Check sheet for the modelled part. Datum: model origin and axes. Units: mm. A direction names the side the tool comes from. Coordinates: 2 decimals unless noted, no trailing zeros. Order: outer loops, then holes, each group sorted by start corner. A loop starts at its lowest first (then second) coordinate and runs counter-clockwise, first axis right, second up. Notation, with made-up numbers: M 17.25,35.25 L 25.25,35.25 A19 cw 25.25,69.25 Z; hole C 36,16.25 d5. An arc over 180 degrees is marked long. Answer in a Markdown table with one row per item. Add a question column.
from build123d import *

# Parameters (mm, degrees)
SKETCH1_R                = 152.4
SKETCH1_R_2              = 133.35
BOSS_EXTRUDE1_DEPTH      = 38.1
SKETCH2_R                = 152.4
SKETCH2_R_2              = 139.7
CUT_EXTRUDE1_DEPTH       = 31.75
BOSS_EXTRUDE2_DEPTH      = 38.1
FILLET1_R                = 2.54
HOLE1_D                  = 8
HOLE1_DEPTH              = 81.182271537
CIRPATTERN1_COUNT        = 3
FILLET1_OF_CIRPATTERN1_R = 2.54
CIRPATTERN2_COUNT        = 16


with BuildPart() as part:
    # Sketch1 → Boss-Extrude1 (new body)
    with BuildSketch(Plane(origin=(0, 0, 0), x_dir=(1, 0, 0), z_dir=(0, 1, 0))):
        Circle(SKETCH1_R)
        Circle(SKETCH1_R_2, mode=Mode.SUBTRACT)
    extrude(amount=BOSS_EXTRUDE1_DEPTH)

    # Sketch2 → Cut-Extrude1 (cut)
    with BuildSketch(Plane(origin=(0, 38.1, 0), x_dir=(1, 0, 0), z_dir=(0, 1, 0))):
        Circle(SKETCH2_R)
        Circle(SKETCH2_R_2, mode=Mode.SUBTRACT)
    extrude(amount=-CUT_EXTRUDE1_DEPTH, mode=Mode.SUBTRACT)

    # Sketch3 → Boss-Extrude2 (add, through all)
    with BuildSketch(Plane(origin=(0, 38.1, 0), x_dir=(1, 0, 0), z_dir=(0, 1, 0))):
        with BuildLine():
            Line((127, 25.4), (127, -25.4))
            Line((127, -25.4), (130.908603613, -25.4))
            ThreePointArc((130.908603613, -25.4), (133.35, 0), (130.908603613, 25.4))
            Line((130.908603613, 25.4), (127, 25.4))
        make_face()
    boss_extrude2 = extrude(amount=-BOSS_EXTRUDE2_DEPTH)

    # Fillet1
    fillet1_edges = [part.edges().sort_by_distance(p)[0] for p in [
        (130.908603613, 19.05, -25.4),
        (130.908603613, 19.05, 25.4),
    ]]
    fillet(fillet1_edges, radius=FILLET1_R)

    # Hole1
    with Locations(Plane(origin=(127, 0, -417.943859866), x_dir=(0, 0, 1), z_dir=(-1, 0, 0))):
        with Locations((400.481359866, 19.05), (435.406359866, 19.05)):
            hole1 = Hole(HOLE1_D / 2, depth=HOLE1_DEPTH)

    # CirPattern1: Boss-Extrude2, Hole1 ×3 about axis
    cirpattern1_axis = Axis((0, 0, 0), (0, 1, 0))
    for i in range(1, CIRPATTERN1_COUNT):
        add(boss_extrude2.rotate(cirpattern1_axis, i * 360 / CIRPATTERN1_COUNT))
        add(hole1.rotate(cirpattern1_axis, i * 360 / CIRPATTERN1_COUNT), mode=Mode.SUBTRACT)

    # Fillet1 of CirPattern1
    fillet1_of_cirpattern1_edges = [part.edges().sort_by_distance(p)[0] for p in [
        (-87.451347063, 19.05, -100.670176303),
        (-43.457256551, 19.05, -126.070176303),
        (-43.457256551, 19.05, 126.070176303),
        (-87.451347063, 19.05, 100.670176303),
    ]]
    fillet(fillet1_of_cirpattern1_edges, radius=FILLET1_OF_CIRPATTERN1_R)

    # Sketch8 → CBORE for #10 Socket Head Cap Screw1 (revolve, cut)
    with BuildSketch(Plane(origin=(146.05, 6.35, 0), x_dir=(0, 0, 1), z_dir=(1, 0, 0))):
        Polygon((0, 0), (0, 9.407816902), (2.5527, 7.874), (2.5527, 4.826), (4.7625, 4.826), (4.7625, 0), align=None)
    cbore_for_10_socket_head_cap_screw1 = revolve(axis=Axis((146.05, 12.7, 0), (0, -1, 0)), mode=Mode.SUBTRACT)

    # CirPattern2: CBORE for #10 Socket Head Cap Screw1 ×16 about axis
    cirpattern2_axis = Axis((0, 0, 0), (0, 1, 0))
    for i in range(1, CIRPATTERN2_COUNT):
        add(cbore_for_10_socket_head_cap_screw1.rotate(cirpattern2_axis, i * 360 / CIRPATTERN2_COUNT), mode=Mode.SUBTRACT)


solid = part.part
1. Go/stop test with flat-tipped pins: pin 1 Ø7.5 at (x, z) = (135, -56) entering from +Y; pin 2 Ø10.5 at (y, z) = (19.05, -17.46) entering from -X; pin 3 Ø4 at (x, z) = (55.89, -134.93) entering from +Y; pin 4 Ø2 at (y, z) = (23.5, 19.5) entering from +X. Record where each tip stops, or that it passes through.
2. Release check for a two-part mould opening along Z. For faces 5 (the cylindrical face through (-110.86, 22.45, 85.01)), 6 (the flat face through (67, 6.35, 123)), 7 (the cylindrical face through (-1.03, 3.97, -150.7)) record: released by +Z, released by -Z, zero draft, split by the parting line, or undercut.
3. Section check A-A on x = 35.5. Enter the section's corners in (y, z).
4. Scan lines: line 1 (Y direction, x = -48, z = 119); line 2 (X direction, y = 30.5, z = -18); line 3 (X direction, y = 17.5, z = -5). Record each from-to range of solid material in increasing order.
5. Section check B-B on y = 11. Enter the section's corners in (x, z), then the cut area to 3 significant figures.
6. Set-up check for faces 1 (the cylindrical face through (-133.34, 18.78, -1.55)), 2 (the cylindrical face through (98.515, 3.971, -103.479)), 3 (the cylindrical face through (133.109, 17.518, 13.768)), 4 (the flat face through (-80, 0, 101)): record each of +Z, -Z, +X, -X, +Y, -Y from which the full face is reachable in a straight line by a thin tool's end or side.
Result sheet:
| question | item | result |
|---|---|---|
| 1 | pin 1 | y = 1.52 |
| 1 | pin 2 | x = -139.17 |
| 1 | pin 3 | through |
| 1 | pin 4 | x = 138.47 |
| 2 | face 5 | split by the parting line |
| 2 | face 6 | zero draft |
| 2 | face 7 | undercut |
| 3 | outline | M 0,-148.21 L 6.35,-148.21 L 6.35,-135.11 L 38.1,-135.11 L 38.1,-128.54 L 0,-128.54 Z; M 0,128.54 L 38.1,128.54 L 38.1,135.11 L 6.35,135.11 L 6.35,148.21 L 0,148.21 Z |
| 4 | line 1 | 0 to 15.08, 23.02 to 38.1 |
| 4 | line 2 | -138.54 to -132.13, 127 to 138.54 |
| 4 | line 3 | -139.61 to -133.26, 127 to 139.61 |
| 5 | outline | C 0,0 d279.4; hole M -89.8,-98.58 A2.54 ccw -85.89,-97.97 L -85.5,-97.29 L -41.5,-122.69 L -41.9,-123.37 A2.54 ccw -40.47,-127.06 A133.35 ccw 130.27,-28.48 A2.54 ccw 127.79,-25.4 L 127,-25.4 L 127,25.4 L 127.79,25.4 A2.54 ccw 130.27,28.48 A133.35 ccw -40.47,127.06 A2.54 ccw -41.9,123.37 L -41.5,122.69 L -85.5,97.29 L -85.89,97.97 A2.54 ccw -89.8,98.58 A133.35 ccw Z |
| 5 | area | 6,300 mm^2 |
| 6 | face 1 | +Y, -Y |
| 6 | face 2 | +Y |
| 6 | face 3 | +X |
| 6 | face 4 | +Z, -Z, +X, -X, -Y |
